The model under review builds one solid part; all positions refer to its coordinate system, in mm. Face numbers are marked on the shaded views. A direction names the side the tool comes from. Give positions to 0.01 mm unless a question says otherwise; leave off trailing zeros. Order: outer loops, then holes, each group sorted by start corner. A loop starts at its lowest first (then second) coordinate and runs counter-clockwise, first axis right, second up. Notation, with made-up numbers: (71.5, -23) -> (85.5, -23) arc R32 cw to (85.5, 10) -> close; hole circle Ø7 at (55.5, -28.75). An arc over 180 degrees is marked (long way). Use one line per item in the form item = value.
```python
from build123d import *

# Parameters (mm, degrees)
F0_R      = 20
F1_DEPTH  = 6
F2_SIZE   = 1.5
F4_R      = 12
F5_DEPTH  = 4.25
F7_R      = 12.75
F8_DEPTH  = 5.5
F10_R     = 12
F11_DEPTH = 4.25
F13_R     = 20
F14_DEPTH = 6
F15_SIZE  = 1.5


with BuildPart() as f1:
    # F0 (on Top) → F1 (new body)
    with BuildSketch(Plane.XY):
        Circle(F0_R)
    extrude(amount=F1_DEPTH)

    # F2
    f2_edges = [f1.edges().sort_by_distance(p)[0] for p in [
        (-20, 0, 6),
    ]]
    chamfer(f2_edges, length=F2_SIZE)

    # F4 (on offset) → F5 (join)
    with BuildSketch(Plane.XY.offset(6)):
        Circle(F4_R)
    extrude(amount=F5_DEPTH)

    # F7 (on offset) → F8 (join)
    with BuildSketch(Plane.XY.offset(10.25)):
        Circle(F7_R)
    extrude(amount=F8_DEPTH)

    # F10 (on offset) → F11 (join)
    with BuildSketch(Plane.XY.offset(15.75)):
        Circle(F10_R)
    extrude(amount=F11_DEPTH)

    # F13 (on offset) → F14 (join)
    with BuildSketch(Plane.XY.offset(20)):
        Circle(F13_R)
    extrude(amount=F14_DEPTH)

    # F15
    f15_edges = [f1.edges().sort_by_distance(p)[0] for p in [
        (-20, 0, 20),
    ]]
    chamfer(f15_edges, length=F15_SIZE)


solid = f1.part
```
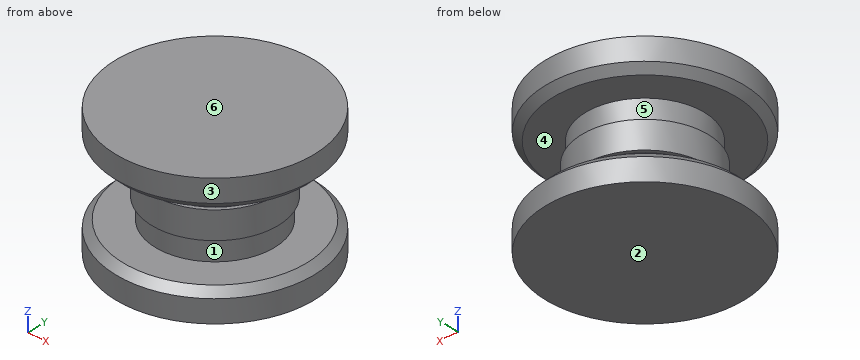
1. For pin 1 Ø4 at (y, z) = (13, 8.5) entering from +X; pin 2 Ø8 at (x, z) = (13, 8) entering from -Y; pin 3 Ø8 at (y, z) = (-10.5, 20.5) entering from -X, all flat-tipped, find the tip position at first contact; note any pin that passes through.
Values:
pin_1 = 4.8
pin_2 = -16.66
pin_3 = -18.87
2. For L1, parallel to Z at x = 4, y = -13.5; L2, parallel to Z at x = 7, y = -10.5; L3, parallel to Z at x = -17, y = -7.5, list the stretches that pass through material, from the lowest coordinate up.
Values:
L1 = 0 to 6, 20 to 26
L2 = 0 to 6, 10.25 to 15.75, 20 to 26
L3 = 0 to 5.92, 20.08 to 26
3. Add section A-A on x = 0. Give the boundary of the cut face in (y, z), then the cut area to 3 significant figures.
Values:
outline = (-20, 0) -> (20, 0) -> (20, 4.5) -> (18.5, 6) -> (12, 6) -> (12, 10.25) -> (12.75, 10.25) -> (12.75, 15.75) -> (12, 15.75) -> (12, 20) -> (18.5, 20) -> (20, 21.5) -> (20, 26) -> (-20, 26) -> (-20, 21.5) -> (-18.5, 20) -> (-12, 20) -> (-12, 15.75) -> (-12.75, 15.75) -> (-12.75, 10.25) -> (-12, 10.25) -> (-12, 6) -> (-18.5, 6) -> (-20, 4.5) -> close
area = 820 mm^2
4. Add section C-C on z = 11.5. Give the boundary of the cut face in (x, y), then the cut area to 3 significant figures.
Values:
outline = circle Ø25.5 at (0, 0)
area = 511 mm^2
5. The part is to be moulded in two halves that separate along Z. For the marked faces 1, 2, 3 and 4, say which applies: +Z half, -Z half, draft (parallel to the pull), parting line (faces both ways), or undercut.
Values:
face_1 = undercut
face_2 = -Z half
face_3 = draft
face_4 = undercut
6. Add section D-D on z = 3.5. Give the boundary of the cut face in (x, y).
Values:
outline = circle Ø40 at (0, 0)
7. Tool access review of the marked faces 5 and 6: name each direction out of +Z, -Z, +X, -X, +Y, -Y from which nothing blocks a thin tool from reaching the whole face with its end or side.
Values:
face_5 = none
face_6 = +Z, +X, -X, +Y, -Y
